from build123d import *

# Parameters (mm, degrees)
SALIENTE_EXTRUIR1_DEPTH = 20
SALIENTE_EXTRUIR2_DEPTH = 3
SALIENTE_EXTRUIR3_DEPTH = 3
SALIENTE_EXTRUIR4_DEPTH = 1.5
CROQUIS5_R              = 2.5
CORTAR_EXTRUIR1_DEPTH   = 38.238203332
CROQUIS6_R              = 2.5
CORTAR_EXTRUIR2_DEPTH   = 41.360446068


with BuildPart() as part:
    # Croquis1 → Saliente-Extruir1 (new, symmetric)
    with BuildSketch(Plane(origin=(0, 0, 0), x_dir=(1, 0, 0), z_dir=(0, 1, 0))):
        Polygon((-19.515220747, 8.373775577), (6.484779253, 8.373775577), (6.484779253, 12.373775577), (-23.515220747, 12.373775577), (-23.515220747, -17.626224423), (-19.515220747, -17.626224423), align=None)
    extrude(amount=SALIENTE_EXTRUIR1_DEPTH, both=True)

    # Croquis2 → Saliente-Extruir2 (add)
    with BuildSketch(Plane.XZ.offset(20)):
        Polygon((-6.515220747, -8.373775577), (-19.515220747, -8.373775577), (-19.515220747, 4.626224423), align=None)
    extrude(amount=-SALIENTE_EXTRUIR2_DEPTH)

    # Croquis3 → Saliente-Extruir3 (add)
    with BuildSketch(Plane(origin=(0, 20, 0), x_dir=(1, 0, 0), z_dir=(0, 1, 0))):
        Polygon((-6.515220747, 8.373775577), (-19.515220747, -4.626224423), (-19.515220747, 8.373775577), align=None)
    extrude(amount=-SALIENTE_EXTRUIR3_DEPTH)

    # Croquis4 → Saliente-Extruir4 (add, symmetric)
    with BuildSketch(Plane(origin=(0, 0, 0), x_dir=(1, 0, 0), z_dir=(0, 1, 0))):
        Polygon((-13.015220747, 8.373775577), (-19.515220747, 1.873775577), (-19.515220747, 8.373775577), align=None)
    extrude(amount=SALIENTE_EXTRUIR4_DEPTH, both=True)

    # Croquis5 → Cortar-Extruir1 (cut, through all)
    with BuildSketch(Plane(origin=(-19.515220747, 0, 0), x_dir=(0, 0, -1), z_dir=(1, 0, 0))):
        with Locations((-4.626224423, -8.5)):
            Circle(CROQUIS5_R)
        with Locations((-4.626224423, 8.5)):
            Circle(CROQUIS5_R)
    extrude(amount=-CORTAR_EXTRUIR1_DEPTH, mode=Mode.SUBTRACT)

    # Croquis6 → Cortar-Extruir2 (cut, through all)
    with BuildSketch(Plane.XY.offset(-8.373775577)):
        with Locations((-6.515220747, -8.5)):
            Circle(CROQUIS6_R)
        with Locations((-6.515220747, 8.5)):
            Circle(CROQUIS6_R)
    extrude(amount=-CORTAR_EXTRUIR2_DEPTH, mode=Mode.SUBTRACT)


solid = part.part
Geometry check sheet. Reference: the model listing, model coordinates, mm. A direction names the side the tool comes from. Coordinates: 2 decimals unless noted, no trailing zeros. Order: outer loops, then holes, each group sorted by start corner. A loop starts at its lowest first (then second) coordinate and runs counter-clockwise, first axis right, second up. Notation, with made-up numbers: (27, 40) -> (53, 40) arc R24 ccw to (53, 64) -> close; hole circle Ø8 at (16, 60.25). An arc over 180 degrees is marked (long way). Use a Markdown table: item, result. Add a question column.
1. Material ranges on L1, parallel to X at y = 13, z = -1.75; L2, parallel to Z at x = 0, y = -15; L3, parallel to Y at x = -17, z = 0, recorded low to high.
2. Cross-section at B-B (z = 11). Enter the section's corners in (x, y), and give its area (3 significant figures).
3. Set-up check for faces 4 (the face through (-16, 17, -5)), 5 (the face through (-22, 0, 17.626)): record each of +Z, -Z, +X, -X, +Y, -Y from which the full face is reachable in a straight line by a thin tool's end or side.
4. Mould release check, pull along Z, two halves, no side actions. Record for faces 1 (the face through (-18, -1.5, -7)), 2 (the face through (-7, 0, -8.374)), 3 (the face through (-21.487, 6.282, 3.473)): pulls with the +Z half, pulls with the -Z half, needs draft (parallel to the pull), parting line crosses it, or undercut.
5. Go/stop test with flat-tipped pins: pin 1 Ø8 at (y, z) = (-1, -0.5) entering from +X; pin 2 Ø4.5 at (y, z) = (-8.5, 4.63) entering from +X; pin 3 Ø8 at (x, y) = (-6.52, 8.5) entering from +Z. Record where each tip stops, or that it passes through.
6. Cross-section at A-A (y = 8.5). Enter the section's corners in (x, z), and give its area (3 significant figures).
7. Cross-section at D-D (y = -16). Enter the section's corners in (x, z).
8. Cross-section at C-C (x = 2). Enter the section's corners in (y, z).
Filled sheet:
| question | item | result |
|---|---|---|
| 1 | L1 | -23.52 to -19.52 |
| 1 | L2 | -12.37 to -8.37 |
| 1 | L3 | -20 to -17, 17 to 20 |
| 2 | outline | (-23.52, -20) -> (-19.52, -20) -> (-19.52, 20) -> (-23.52, 20) -> close |
| 2 | area | 160 mm2 |
| 3 | face 4 | +Z, +X |
| 3 | face 5 | +Z, +X, -X, +Y, -Y |
| 4 | face 1 | needs draft |
| 4 | face 2 | pulls with the +Z half |
| 4 | face 3 | undercut |
| 5 | pin 1 | x = -16.89 |
| 5 | pin 2 | through |
| 5 | pin 3 | z = -8.37 |
| 6 | outline | (-23.52, -12.37) -> (-9.02, -12.37) -> (-9.02, -8.37) -> (-19.52, -8.37) -> (-19.52, 2.13) -> (-23.52, 2.13) -> close; (-23.52, 7.13) -> (-19.52, 7.13) -> (-19.52, 17.63) -> (-23.52, 17.63) -> close; (-4.02, -12.37) -> (6.48, -12.37) -> (6.48, -8.37) -> (-4.02, -8.37) -> close |
| 6 | area | 184 mm2 |
| 7 | outline | (-23.52, -12.37) -> (6.48, -12.37) -> (6.48, -8.37) -> (-19.52, -8.37) -> (-19.52, 17.63) -> (-23.52, 17.63) -> close |
| 8 | outline | (-20, -12.37) -> (20, -12.37) -> (20, -8.37) -> (-20, -8.37) -> close |
